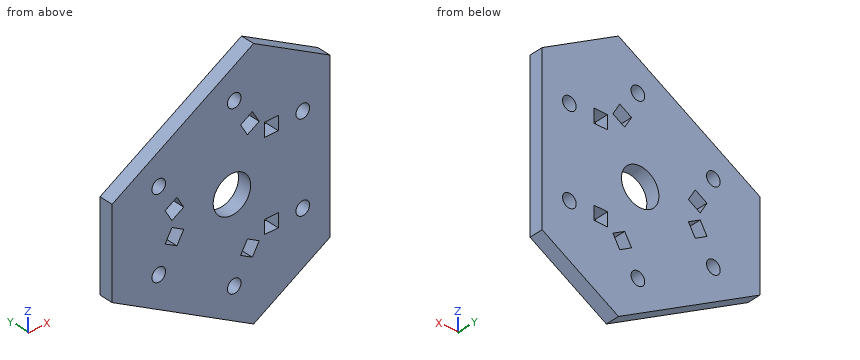
```python
from build123d import *

# Parameters (mm, degrees)
SKETCH2_R           = 1.5875
SKETCH2_R_2         = 4.365625
SKETCH2_W           = 3.175
SKETCH2_H           = 3.175
BOSS_EXTRUDE2_DEPTH = 3.175


with BuildPart() as part:
    # Sketch2 → Boss-Extrude2 (new body)
    with BuildSketch(Plane(origin=(0, 0, 0), x_dir=(1, 0, 0), z_dir=(0, 1, 0))):
        Polygon((22.868144039, 19.05), (22.868144039, -19.05), (5.063711923, -29.329393675), (-27.931855961, -10.279393675), (-27.931855961, 10.279393675), (5.063711923, 29.329393675), align=None)
        with Locations((16.518144039, 10.16)):
            Circle(SKETCH2_R, mode=Mode.SUBTRACT)
        with Locations((16.518144039, -10.16)):
            Circle(SKETCH2_R, mode=Mode.SUBTRACT)
        with Locations((0.539746083, -19.385132361)):
            Circle(SKETCH2_R, mode=Mode.SUBTRACT)
        Circle(SKETCH2_R_2, mode=Mode.SUBTRACT)
        with Locations((-17.057890122, -9.225132361)):
            Circle(SKETCH2_R, mode=Mode.SUBTRACT)
        with Locations((-17.057890122, 9.225132361)):
            Circle(SKETCH2_R, mode=Mode.SUBTRACT)
        with Locations((0.539746083, 19.385132361)):
            Circle(SKETCH2_R, mode=Mode.SUBTRACT)
        with Locations((9.215644039, 10.16)):
            Rectangle(SKETCH2_W, SKETCH2_H, mode=Mode.SUBTRACT)
        with Locations((9.215644039, -10.16)):
            Rectangle(SKETCH2_W, SKETCH2_H, mode=Mode.SUBTRACT)
        Polygon((3.609930755, -10.892416521), (2.022430755, -13.642047178), (4.772061412, -15.229547178), (6.359561412, -12.479916521), align=None, mode=Mode.SUBTRACT)
        Polygon((-11.238074793, -2.319916521), (-12.825574793, -5.069547178), (-15.57520545, -3.482047178), (-13.98770545, -0.732416521), align=None, mode=Mode.SUBTRACT)
        Polygon((-11.238074793, 2.319916521), (-12.825574793, 5.069547178), (-15.57520545, 3.482047178), (-13.98770545, 0.732416521), align=None, mode=Mode.SUBTRACT)
        Polygon((3.609930755, 10.892416521), (2.022430755, 13.642047178), (4.772061412, 15.229547178), (6.359561412, 12.479916521), align=None, mode=Mode.SUBTRACT)
    extrude(amount=BOSS_EXTRUDE2_DEPTH)


solid = part.part
```
Read the model definition and answer for the solid it produces. Units are mm, in the model's axes. Coordinates: 2 decimals unless noted, no trailing zeros. Loops run counter-clockwise (first coordinate to the right, second up) from the corner with the lowest first, then second, coordinate; pieces in that order, holes last.
(1) The part is cut by section B-B (x = 8.5). Determine the outline of the cut face in (y, z) (1 decimal).
Solution:
outline: (0, -27.3) - (3.2, -27.3) - (3.2, -11.7) - (0, -11.7) - close; (0, -8.6) - (3.2, -8.6) - (3.2, 8.6) - (0, 8.6) - close; (0, 11.7) - (3.2, 11.7) - (3.2, 27.3) - (0, 27.3) - close
(2) The part is cut by section C-C (x = 0). Determine the outline of the cut face in (y, z) (3 decimals), and give its area (3 significant figures).
Solution:
outline: (0, -26.406) - (3.175, -26.406) - (3.175, -20.878) - (0, -20.878) - close; (0, -17.892) - (3.175, -17.892) - (3.175, -4.366) - (0, -4.366) - close; (0, 4.366) - (3.175, 4.366) - (3.175, 17.892) - (0, 17.892) - close; (0, 20.878) - (3.175, 20.878) - (3.175, 26.406) - (0, 26.406) - close
area: 121 mm2
(3) Consider line 1 along X through (y, z) = (1.1, 0); line 2 along Z through (x, y) = (4, 2); line 3 along Z through (x, y) = (8, 2.4). Determine where each line is inside the solid, lowest interval first.
Solution:
line 1: x = -27.93 to -4.37, 4.37 to 22.87
line 2: z = -28.72 to -14.78, -11.12 to -1.75, 1.75 to 11.12, 14.78 to 28.72
line 3: z = -27.63 to -11.75, -8.57 to 8.57, 11.75 to 27.63
(4) Flat-ended cylindrical pins translate along their axes: pin 1 Ø1 at (x, y) = (9, 2) entering from -Z; pin 2 Ø5 at (x, z) = (0.54, 19.39) entering from +Y (3 decimals); pin 3 Ø2.5 at (x, z) = (16.52, 10.16) entering from -Y; pin 4 Ø1 at (x, y) = (2.5, 1) entering from +Z. Find the tip coordinate at first contact, or state that the pin passes through.
Solution:
pin 1: stops at z = -27.35
pin 2: stops at y = 3.175
pin 3: passes through
pin 4: stops at z = 28.14
(5) The part is cut by section A-A (z = 0). Determine the outline of the cut face in (x, y) (3 decimals), and give its area (3 significant figures).
Solution:
outline: (-27.932, 0) - (-4.366, 0) - (-4.366, 3.175) - (-27.932, 3.175) - close; (4.366, 0) - (22.868, 0) - (22.868, 3.175) - (4.366, 3.175) - close
area: 134 mm2
(6) The part is cut by section D-D (z = -14.5). Determine the outline of the cut face in (x, y) (3 decimals), and give its area (3 significant figures).
Solution:
outline: (-20.622, 0) - (3.508, 0) - (3.508, 3.175) - (-20.622, 3.175) - close; (5.193, 0) - (22.868, 0) - (22.868, 3.175) - (5.193, 3.175) - close
area: 133 mm2
